CAD build for the part. Positions are in the model's coordinates, mm. A direction names the side the tool comes from. Coordinates: 2 decimals unless noted, no trailing zeros. Loops run counter-clockwise (first coordinate to the right, second up) from the corner with the lowest first, then second, coordinate; pieces in that order, holes last.
1) Two-plate mould, pull along Y, no slides. Class faces 6 (the cylindrical face through (-1.115, 1.216, -40.021)), 7 (the conical face through (-0.1, -0.3, -34.1)), 8 (the flat face through (4, 0, -42)), 9 (the cylindrical face through (5, 0, 1)): +Y half, -Y half, draft (parallel to the pull), parting line (faces both ways), or undercut.
2) Saw through at B-B, the plane x = -2.5. Write the cut outline in (y, z).
3) Saw through at A-A, the plane z = -7. Write the cut outline in (x, y), and give its area (3 significant figures).
4) Saw through at C-C, the plane y = 4.25. Write the cut outline in (x, z).
5) Wall check: line 1 along X through (y, z) = (0, -37); line 2 along X through (y, z) = (0, 42.5); line 3 along X through (y, z) = (3, 29). Give the ranges that are in metal, low to high.
6) Pin check, flat tips, straight feed: pin 1 Ø4 at (x, y) = (0, 0) entering from -Z; pin 2 Ø2 at (x, z) = (-2, -3) entering from -Y; pin 3 Ø0.8 at (x, y) = (4.5, -1) entering from +Z; pin 4 Ø1.5 at (y, z) = (-2, 22.5) entering from -X. Stop position of each tip, or through.
7) Which spindle directions (+Z, -Z, +X, -X, +Y, -Y) get a long thin tool onto all of the face, cutting with end or side? Do faces 1 (the flat face through (4, 0, 42)), 2 (the cylindrical face through (-1.115, 1.216, 40.021)), 3 (the flat face through (-4, 0, 42)), 4 (the flat face through (-4, 0, -42)), 5 (the flat face through (-2, 0, -45)). Say none if no direction does.
```python
from build123d import *

# Parameters (mm, degrees)
SKETCH_1_R          = 5
EXTRUDE_1_DEPTH     = 45
CUT_EXTRUDE_1_DEPTH = 6


with BuildPart() as part:
    # 草图1 → 凸台-拉伸1 (new, symmetric)
    with BuildSketch(Plane.XY):
        with Locations(Location((0, 0, 0), (0, 0, 180))):
            Circle(SKETCH_1_R)
    extrude(amount=EXTRUDE_1_DEPTH, both=True)

    # 草图2 → 切除-拉伸1 (cut)
    with BuildSketch(Plane.XY.offset(45)):
        with BuildLine():
            Line((-4, -3), (-4, 3))
            ThreePointArc((-4, 3), (-5, 0), (-4, -3))
        make_face()
        with BuildLine():
            Line((4, -3), (4, 3))
            ThreePointArc((4, 3), (5, 0), (4, -3))
        make_face()
    cut_extrude_1 = extrude(amount=-CUT_EXTRUDE_1_DEPTH, mode=Mode.SUBTRACT)

    # 草图3 → M4 螺纹孔1 (revolve, cut)
    with BuildSketch(Plane(origin=(0, 0, 45), x_dir=(0, -1, 0), z_dir=(1, 0, 0))):
        Polygon((0, 0), (0, 11.091420021), (1.65, 10.1), (1.65, 0), align=None)
    hole_wizard_m4_1 = revolve(axis=Axis((0, 0, 51.35), (0, 0, -1)), mode=Mode.SUBTRACT)

    # 镜向1: 切除-拉伸1, M4 螺纹孔1 across plane
    add(cut_extrude_1.mirror(Plane.XY), mode=Mode.SUBTRACT)
    add(hole_wizard_m4_1.mirror(Plane.XY), mode=Mode.SUBTRACT)


solid = part.part
```
Data:
1. face 6: undercut
1. face 7: undercut
1. face 8: draft
1. face 9: parting line
2. outline: (-4.33, -45) - (4.33, -45) - (4.33, 45) - (-4.33, 45) - close
3. outline: circle Ø10 at (0, 0)
3. area: 78.5 mm2
4. outline: (-2.63, -45) - (2.63, -45) - (2.63, 45) - (-2.63, 45) - close
5. line 1: x = -5 to -1.65, 1.65 to 5
5. line 2: x = -4 to -1.65, 1.65 to 4
5. line 3: x = -4 to 4
6. pin 1: stops at z = -45
6. pin 2: stops at y = -4.9
6. pin 3: stops at z = 39
6. pin 4: stops at x = -4.84
7. face 1: +Z, +X, +Y, -Y
7. face 2: +Z
7. face 3: +Z, -X, +Y, -Y
7. face 4: -Z, -X, +Y, -Y
7. face 5: -Z, +X, -X, +Y, -Y
